Could you check a few things on this model? Use its own coordinates, in mm. A direction names the side the tool comes from. Coordinates: 2 decimals unless noted, no trailing zeros. Order: outer loops, then holes, each group sorted by start corner. A loop starts at its lowest first (then second) coordinate and runs counter-clockwise, first axis right, second up. Notation, with made-up numbers: (-6, 7) - (15, 7) arc R7 cw to (15, 19) - close; hole circle Ø9 at (63, 45). An arc over 180 degrees is marked (long way). Answer as a JSON object with one key per item and string values. Group by question number.
(1) Imagine slicing it at D-D, the plane z = 36. Write out the boundary of the cut face in (x, y), and give its area (3 significant figures).
(2) Imagine slicing it at C-C, the plane y = 14. Write out the boundary of the cut face in (x, z), and give its area (3 significant figures).
(3) Imagine slicing it at A-A, the plane y = 0. Write out the boundary of the cut face in (x, z).
(4) Will this pin go through, and if not, where does the flat tip stop? P1, Ø2, axis at x = 1.5, y = -34, coming from the +Z side.
(5) Please list where these lines run through material, in increasing order: probe 1 along X at (y, z) = (-2.5, 27); probe 2 along Y at (x, z) = (-16.5, 57.5); probe 3 along Y at (x, z) = (18, 63).
(6) Imagine slicing it at B-B, the plane x = -12. Write out the boundary of the cut face in (y, z), and give its area (3 significant figures).
(7) We'd pull the mould along X, two halves only. Please class faces 1 (the flat face through (0, 34, 68.707)), 2 (the flat face through (33.363, 0, 26)), 3 (the flat face through (30.823, 7, 34)), 4 (the flat face through (0, -32.169, 34)): pulls with the +X half, pulls with the -X half, needs draft (parallel to the pull), parting line crosses it, or undercut.
(8) Which directions (+Z, -Z, +X, -X, +Y, -Y) give clear straight access to the entire face, cutting with the end or side of a thin tool? Please do faces 5 (the flat face through (27.94, -33, 64)), 6 (the flat face through (-30.823, 7, 34)), 7 (the cylindrical face through (-32.111, 4.251, 37.064)).
from build123d import *

# Parameters (mm, degrees)
SKETCH1_W               = 66.7258
SKETCH1_H               = 69.4182
SKETCH1_W_2             = 61.6458
SKETCH1_H_2             = 64.3382
EXTRUDE_THIN1_DEPTH     = 68.707
F_3_8_CLEARANCE_HOLE1_D = 10.0838
SKETCH4_W               = 55.88
SKETCH4_H               = 8.89
CUT_EXTRUDE1_DEPTH      = 3.54


with BuildPart() as part:
    # Sketch1 → Extrude-Thin1 (new body)
    with BuildSketch(Plane.XY):
        Rectangle(SKETCH1_W, SKETCH1_H)
        Rectangle(SKETCH1_W_2, SKETCH1_H_2, mode=Mode.SUBTRACT)
    extrude(amount=EXTRUDE_THIN1_DEPTH)

    # 3/8 Clearance Hole1 (through all)
    with Locations(Plane(origin=(33.3629, 0, 0), x_dir=(0, 0, -1), z_dir=(1, 0, 0))):
        with Locations((-34.3535, 0)):
            Hole(F_3_8_CLEARANCE_HOLE1_D / 2)

    # Sketch4 → Cut-Extrude1 (cut, through all)
    with BuildSketch(Plane(origin=(0, -32.1691, 0), x_dir=(1, 0, 0), z_dir=(0, 1, 0))):
        with Locations((0, -64.262)):
            Rectangle(SKETCH4_W, SKETCH4_H)
    extrude(amount=-CUT_EXTRUDE1_DEPTH, mode=Mode.SUBTRACT)


solid = part.part
Result set:
{
 "1": {"outline": "(-33.36, -34.71) - (33.36, -34.71) - (33.36, -4.77) - (30.82, -4.77) - (30.82, -32.17) - (-30.82, -32.17) - (-30.82, -4.77) - (-33.36, -4.77) - close; (-33.36, 4.77) - (-30.82, 4.77) - (-30.82, 32.17) - (30.82, 32.17) - (30.82, 4.77) - (33.36, 4.77) - (33.36, 34.71) - (-33.36, 34.71) - close", "area": "617 mm^2"},
 "2": {"outline": "(-33.36, 0) - (-30.82, 0) - (-30.82, 68.71) - (-33.36, 68.71) - close; (30.82, 0) - (33.36, 0) - (33.36, 68.71) - (30.82, 68.71) - close", "area": "349 mm^2"},
 "3": {"outline": "(-33.36, 0) - (-30.82, 0) - (-30.82, 29.31) - (-33.36, 29.31) - close; (-33.36, 39.4) - (-30.82, 39.4) - (-30.82, 68.71) - (-33.36, 68.71) - close; (30.82, 0) - (33.36, 0) - (33.36, 29.31) - (30.82, 29.31) - close; (30.82, 39.4) - (33.36, 39.4) - (33.36, 68.71) - (30.82, 68.71) - close"},
 "4": {"P1": "stops at z = 59.82"},
 "5": {"probe 1": "x = -33.36 to -30.82, 30.82 to 33.36", "probe 2": "y = -34.71 to -32.17, 32.17 to 34.71", "probe 3": "y = 32.17 to 34.71"},
 "6": {"outline": "(-34.71, 0) - (-32.17, 0) - (-32.17, 59.82) - (-34.71, 59.82) - close; (32.17, 0) - (34.71, 0) - (34.71, 68.71) - (32.17, 68.71) - close", "area": "326 mm^2"},
 "7": {"face 1": "needs draft", "face 2": "pulls with the +X half", "face 3": "undercut", "face 4": "undercut"},
 "8": {"face 5": "+Z, -Y", "face 6": "+Z, -Z", "face 7": "+X, -X"}
}
